from build123d import *

# Parameters (mm, degrees)
ESQUISSE1_R             = 13
ESQUISSE1_R_2           = 1.25
ESQUISSE1_R_3           = 3
BOSS_EXTRU_1_DEPTH      = 2.7
CHANFREIN1_SIZE         = 1
CHANFREIN1_SIZE2        = 1.191753593
ESQUISSE3_R             = 3.75
ENL_V_MAT_EXTRU_1_DEPTH = 1
ESQUISSE5_R             = 17.5
ESQUISSE5_R_2           = 12.5
ENL_V_MAT_EXTRU_3_DEPTH = 0.5
ESQUISSE7_R             = 4
BOSS_EXTRU_2_DEPTH      = 8
ESQUISSE8_R             = 1.5
ENL_V_MAT_EXTRU_5_DEPTH = 3


with BuildPart() as part:
    # Esquisse1 → Boss.-Extru.1 (new body)
    # profile 1 of 5: a face of its own
    with BuildSketch(Plane.XY):
        with Locations(Location((0, 0, 0), (0, 0, 180))):
            Circle(ESQUISSE1_R)
        with Locations((-5, -5)):
            Circle(ESQUISSE1_R_2, mode=Mode.SUBTRACT)
        with Locations((-5, 5)):
            Circle(ESQUISSE1_R_2, mode=Mode.SUBTRACT)
        with Locations((5, 5)):
            Circle(ESQUISSE1_R_2, mode=Mode.SUBTRACT)
        with Locations((5, -5)):
            Circle(ESQUISSE1_R_2, mode=Mode.SUBTRACT)
        with Locations(Location((0, -8.4, 0), (0, 0, 180))):
            Circle(ESQUISSE1_R_3, mode=Mode.SUBTRACT)
        with Locations(Location((0, 8.4, 0), (0, 0, 180))):
            Circle(ESQUISSE1_R_3, mode=Mode.SUBTRACT)
    # profile 2 of 5: a face of its own
    with BuildSketch(Plane.XY):
        with Locations((5, -5)):
            Circle(ESQUISSE1_R_2)
    # profile 3 of 5: a face of its own
    with BuildSketch(Plane.XY):
        with Locations((5, 5)):
            Circle(ESQUISSE1_R_2)
    # profile 4 of 5: a face of its own
    with BuildSketch(Plane.XY):
        with Locations((-5, -5)):
            Circle(ESQUISSE1_R_2)
    # profile 5 of 5: a face of its own
    with BuildSketch(Plane.XY):
        with Locations((-5, 5)):
            Circle(ESQUISSE1_R_2)
    extrude(amount=BOSS_EXTRU_1_DEPTH)

    # Chanfrein1
    chanfrein1_edges = [part.edges().sort_by_distance(p)[0] for p in [
        (13, 0, 0),
    ]]
    chanfrein1_side = [part.faces().sort_by_distance(p)[0] for p in [
        (13, 0, 1.35),
    ]]
    chamfer(chanfrein1_edges, length=CHANFREIN1_SIZE, length2=CHANFREIN1_SIZE2, reference=chanfrein1_side[0])

    # Esquisse3 → Enl_v. mat.-Extru.1 (cut)
    with BuildSketch(Plane.XY.offset(2.7)):
        with Locations((0, 8.4)):
            Circle(ESQUISSE3_R)
        with Locations((0, -8.4)):
            Circle(ESQUISSE3_R)
    extrude(amount=-ENL_V_MAT_EXTRU_1_DEPTH, mode=Mode.SUBTRACT)

    # Esquisse5 → Enl_v. mat.-Extru.3 (cut)
    with BuildSketch(Plane.XY.offset(2.7)):
        Circle(ESQUISSE5_R)
        Circle(ESQUISSE5_R_2, mode=Mode.SUBTRACT)
    extrude(amount=-ENL_V_MAT_EXTRU_3_DEPTH, mode=Mode.SUBTRACT)

    # Esquisse7 → Boss.-Extru.2 (add)
    with BuildSketch(Plane.XY.offset(2.7)):
        Circle(ESQUISSE7_R)
    extrude(amount=BOSS_EXTRU_2_DEPTH)

    # Esquisse8 → Enl_v. mat.-Extru.5 (cut)
    with BuildSketch(Plane.XY.offset(10.7)):
        Circle(ESQUISSE8_R)
    extrude(amount=-ENL_V_MAT_EXTRU_5_DEPTH, mode=Mode.SUBTRACT)


solid = part.part
Check sheet for the modelled part. Datum: model origin and axes. Units: mm. A direction names the side the tool comes from. Give positions to 0.01 mm unless a question says otherwise; leave off trailing zeros. Order: outer loops, then holes, each group sorted by start corner. A loop starts at its lowest first (then second) coordinate and runs counter-clockwise, first axis right, second up. Notation, with made-up numbers: (-19.75, 6) - (0.25, 6) arc R20 ccw to (0.25, 19) - close; hole circle Ø6 at (58, 70). An arc over 180 degrees is marked (long way). Answer as CSV lines item,"result".
1. Scan lines: probe 1 along Y at (x, z) = (0, 9.55); probe 2 along Y at (x, z) = (0, 1.2); probe 3 along Y at (x, z) = (0, 2.35). Record each from-to range of solid material in increasing order. Write a range as from..to.
Result sheet:
probe 1,"-4..-1.5, 1.5..4"
probe 2,"-13..-11.4, -5.4..5.4, 11.4..13"
probe 3,"-12.5..-12.15, -4.65..4.65, 12.15..12.5"
2. Go/stop test with flat-tipped pins: P1, Ø1, axis at x = -0.5, z = 9, coming from the -Y side; P2, Ø8, axis at x = 0, y = 8.4, coming from the +Z side; P3, Ø1.8, axis at x = 0, y = 0, coming from the +Z side. Record where each tip stops, or that it passes through.
Result sheet:
P1,"y = -4"
P2,"z = 2.7"
P3,"z = 7.7"
3. Section check B-B (z = 8.75). Record the boundary of the cut face in (x, y).
Result sheet:
outline,"circle Ø8 at (0, 0); hole circle Ø3 at (0, 0)"
4. Section check D-D (z = 3.25). Record the boundary of the cut face in (x, y).
Result sheet:
outline,"circle Ø8 at (0, 0)"
5. Mould release check, pull along Y, two halves, no side actions. Record for faces 3 (the face through (0, 0, 0)), 4 (the face through (11.923, 3.755, 2.454)), 5 (the face through (-1.384, -5.738, 0.838)): released by +Y, released by -Y, zero draft, split by the parting line, or undercut.
Result sheet:
face 3,"zero draft"
face 4,"split by the parting line"
face 5,"undercut"
6. Tool access check on faces 1 (the face through (10.316, 7.91, 1.592)), 2 (the face through (-1.5, 0.07, 9.22)). Record the directions out of +Z, -Z, +X, -X, +Y, -Y that give a thin tool (end or side, any length) a straight path to the whole face; none if there is none.
Result sheet:
face 1,"+Z, -Z"
face 2,"+Z"
7. Section check A-A (x = 0). State how many separate pieces and enclosed holes the cut face has, then the cut area to 3 significant figures.
Result sheet:
separate pieces,"3"
enclosed holes,"0"
area,"88.1 mm²"
8. Section check C-C (y = 0). Record the boundary of the cut face in (x, z).
Result sheet:
outline,"(-13, 1) - (-11.81, 0) - (11.81, 0) - (13, 1) - (13, 2.2) - (12.5, 2.2) - (12.5, 2.7) - (4, 2.7) - (4, 10.7) - (1.5, 10.7) - (1.5, 7.7) - (-1.5, 7.7) - (-1.5, 10.7) - (-4, 10.7) - (-4, 2.7) - (-12.5, 2.7) - (-12.5, 2.2) - (-13, 2.2) - close"
